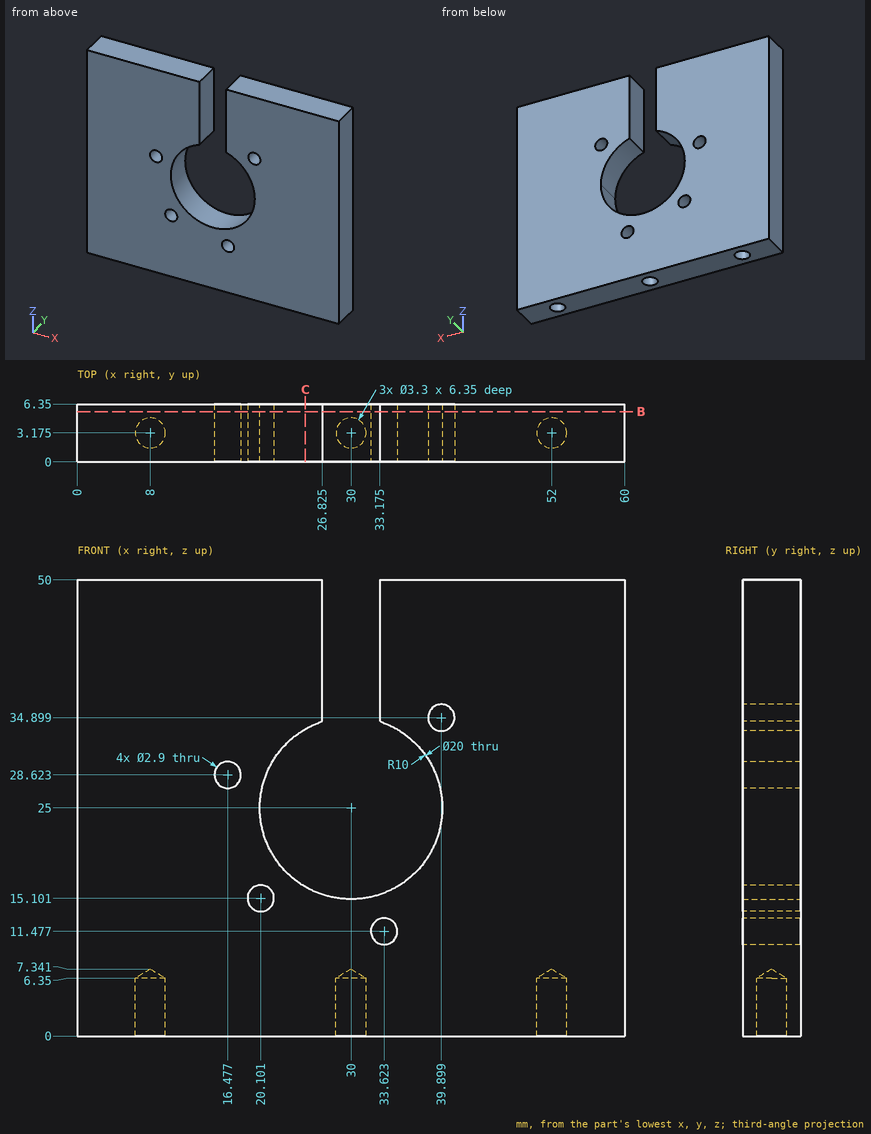
Part print with two shaded views. Sizes in mm from the minimum x, y, z corner. Coordinates: 2 decimals unless noted, no trailing zeros. Loops run counter-clockwise (first coordinate to the right, second up) from the corner with the lowest first, then second, coordinate; pieces in that order, holes last. Notation, with made-up numbers: (70, 19) -> (99, 19) arc R28 ccw to (99, 40) -> close; hole circle Ø1 at (80, 3). An arc over 180 degrees is marked (long way). Answer as a JSON object with one key per item and string values.
Q1. Cut at C-C (x = 25). List the corners of the cut face in (y, z).
Report:
{"outline": "(0, 0) -> (6.35, 0) -> (6.35, 16.34) -> (0, 16.34) -> close; (0, 33.66) -> (6.35, 33.66) -> (6.35, 50) -> (0, 50) -> close"}
Q2. Flat gauge pins, fed straight in: P1, Ø1.7, axis at x = 20.1, z = 15.1, coming from the +Y side; P2, Ø2.5, axis at x = 8, y = 3.175, coming from the -Z side. Where does each tip first touch, or does it go through?
Report:
{"P1": "passes through", "P2": "stops at z = 6.59"}
Q3. Cut at B-B (y = 5.5). State how many separate pieces and enclosed holes the cut face has, and give its area (3 significant figures).
Report:
{"separate pieces": "1", "enclosed holes": "4", "area": "2,560 mm2"}
Q4. Probe probe 1 along X at (y, z) = (0.5, 38.5) (1 decimal); probe 2 along X at (y, z) = (1.25, 34.5) (1 decimal); probe 3 along X at (y, z) = (1.5, 25). List the from-to ranges inside material, lowest first.
Report:
{"probe 1": "x = 0 to 26.8, 33.2 to 60", "probe 2": "x = 0 to 26.8, 33.2 to 38.5, 41.3 to 60", "probe 3": "x = 0 to 20, 40 to 60"}
